Check sheet for the modelled part. Datum: model origin and axes. Units: mm. Face numbers are marked on the shaded views. A direction names the side the tool comes from. Give positions to 0.01 mm unless a question says otherwise; leave off trailing zeros. Order: outer loops, then holes, each group sorted by start corner. A loop starts at its lowest first (then second) coordinate and runs counter-clockwise, first axis right, second up.
```python
from build123d import *

# Parameters (mm, degrees)
BASE_FLANGE1_DEPTH      = 53.975
M4_CLEARANCE_HOLE1_D    = 4.3
F_1_4_CLEARANCE_HOLE1_D = 6.7564
FILLET1_R               = 2.54


# Read off the part's stored shape, not the designer's step: Base-Flange1
with BuildPart() as part:
    # Base-Flange1 outline → Base-Flange1 (new body)
    with BuildSketch(Plane.XY):
        with BuildLine():
            Line((4.98475, 0), (31.75, 0))
            Line((31.75, 0), (31.75, 1.9939))
            Line((31.75, 1.9939), (4.98475, 1.9939))
            ThreePointArc((4.98475, 1.9939), (2.869899683, 2.869899683), (1.9939, 4.98475))
            Line((1.9939, 4.98475), (1.9939, 53.975))
            Line((1.9939, 53.975), (0, 53.975))
            Line((0, 53.975), (0, 4.98475))
            ThreePointArc((0, 4.98475), (1.459999472, 1.459999472), (4.98475, 0))
        make_face()
    extrude(amount=BASE_FLANGE1_DEPTH)

    # M4 Clearance Hole1 (through all)
    with Locations(Plane.ZY):
        with Locations((36.2375, 46.419), (7.237499922, 46.419)):
            Hole(M4_CLEARANCE_HOLE1_D / 2)

    # 1/4 Clearance Hole1 (through all)
    with Locations(Plane(origin=(0, 1.9939, 0), x_dir=(1, 0, 0), z_dir=(0, 1, 0))):
        with Locations((22.225, -44.45), (22.225, -9.525)):
            Hole(F_1_4_CLEARANCE_HOLE1_D / 2)

    # Fillet1
    fillet1_edges = [part.edges().sort_by_distance(p)[0] for p in [
        (0.99695, 53.975, 53.975),
        (0.99695, 53.975, 0),
        (31.75, 0.99695, 53.975),
        (31.75, 0.99695, 0),
    ]]
    fillet(fillet1_edges, radius=FILLET1_R)


solid = part.part
```
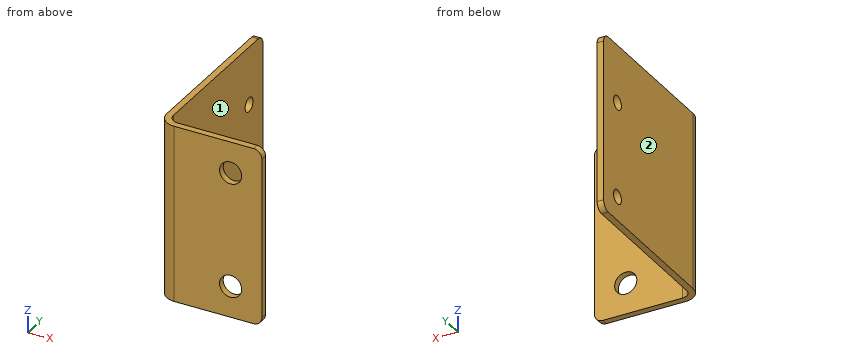
(1) Set-up check for the marked faces 1 and 2: record each of +Z, -Z, +X, -X, +Y, -Y from which the full face is reachable in a straight line by a thin tool's end or side.
Response values:
face 1: +Z, -Z, +X, +Y
face 2: +Z, -Z, -X, +Y, -Y
(2) Material ranges on L1, parallel to X at y = 29.5, z = 29.5; L2, parallel to X at y = 1.6, z = 44.45, recorded low to high.
Response values:
L1: x = 0 to 1.99
L2: x = 1.33 to 18.85, 25.6 to 31.75
(3) Gauge pin test, flat ends, axial feed: pin 1 Ø2 at (x, z) = (28, 37) entering from +Y; pin 2 Ø1.5 at (y, z) = (24, 44.5) entering from +X. Record the tip position at first contact, or that the pin passes through.
Response values:
pin 1: stops at y = 1.99
pin 2: stops at x = 1.99
(4) Cross-section at D-D on y = 4. Enter the section's corners in (x, z) (3 decimals), then the cut area to 3 significant figures.
Response values:
outline: (0.098, 0) - (2.161, 0) - (2.161, 53.975) - (0.098, 53.975) - close
area: 111 mm2
(5) Cross-section at B-B on x = 20.5. Enter the section's corners in (y, z) (3 decimals), then the cut area to 3 significant figures.
Response values:
outline: (0, 0) - (1.994, 0) - (1.994, 6.62) - (0, 6.62) - close; (0, 12.43) - (1.994, 12.43) - (1.994, 41.545) - (0, 41.545) - close; (0, 47.355) - (1.994, 47.355) - (1.994, 53.975) - (0, 53.975) - close
area: 84.5 mm2
